from build123d import *

# Parameters (mm, degrees)
ESQUISSE1_R                                = 30
BOSS_EXTRU_1_DEPTH                         = 15
ESQUISSE2_R                                = 12.5
BOSS_EXTRU_2_DEPTH                         = 124
ESQUISSE4_2_W                              = 230
ESQUISSE4_2_H                              = 40
ENL_V_MAT_EXTRU_1_DEPTH                    = 5
CHAMBRAGE_POUR_VIS_T_TE_HEXAGONALE_2_COUNT = 2
CHAMBRAGE_POUR_VIS_T_TE_HEXAGONALE_2_PITCH = 41
ESQUISSE17_R                               = 6
BOSS_EXTRU_4_DEPTH                         = 83.38
ESQUISSE18_W                               = 10.356322474
ESQUISSE18_H                               = 3
ENL_V_MAT_EXTRU_2_DEPTH                    = 3
ESQUISSE19_W                               = 7.933443835
ESQUISSE19_H                               = 21.9317122
ENL_V_MAT_EXTRU_3_DEPTH                    = 50
BOSS_EXTRU_6_START                         = -10
ESQUISSE21_R                               = 12.5
BOSS_EXTRU_6_DEPTH                         = 10
D_GAGEMENT_M41_D                           = 4.5
D_GAGEMENT_M41_DEPTH                       = 3
D_GAGEMENT_M41_TIP                         = 1.299038106


with BuildPart() as part:
    # Esquisse1 → Boss.-Extru.1 (new body)
    with BuildSketch(Plane.XY):
        Circle(ESQUISSE1_R)
    extrude(amount=BOSS_EXTRU_1_DEPTH)

    # Esquisse2 → Boss.-Extru.2 (add)
    with BuildSketch(Plane(origin=(0, 0, 0), x_dir=(-1, 0, 0), z_dir=(0, 0, -1))):
        with Locations(Location((0, 0, 0), (0, 0, 180))):
            Circle(ESQUISSE2_R)
    extrude(amount=BOSS_EXTRU_2_DEPTH)

    # Esquisse4<2> → Enlèv. mat.-Extru.1 (cut)
    with BuildSketch(Plane.XY.offset(15)):
        Rectangle(ESQUISSE4_2_W, ESQUISSE4_2_H)
    extrude(amount=-ENL_V_MAT_EXTRU_1_DEPTH, mode=Mode.SUBTRACT)

    # Esquisse14 → Chambrage pour vis à tête hexagonale M51 (revolve, cut)
    with BuildSketch(Plane.YZ.offset(-20.5)):
        Polygon((0, 0), (0, 15), (2.75, 15), (2.75, 3.605), (2.775, 3.58), (6.12, 3.58), (6.12, 0), align=None)
    chambrage_pour_vis_t_te_hexagonale_m51 = revolve(axis=Axis((-20.5, 0, -6.35), (0, 0, 1)), mode=Mode.SUBTRACT)

    # Chambrage pour vis _ t_te hexagonale 2: Chambrage pour vis à tête hexagonale M51 ×2
    with Locations(*[(i * CHAMBRAGE_POUR_VIS_T_TE_HEXAGONALE_2_PITCH, 0, 0) for i in range(1, CHAMBRAGE_POUR_VIS_T_TE_HEXAGONALE_2_COUNT)]):
        add(chambrage_pour_vis_t_te_hexagonale_m51, mode=Mode.SUBTRACT)

    # Esquisse17 → Boss.-Extru.4 (add)
    with BuildSketch(Plane(origin=(0, 0, -124), x_dir=(-1, 0, 0), z_dir=(0, 0, -1))):
        Circle(ESQUISSE17_R)
    extrude(amount=BOSS_EXTRU_4_DEPTH)

    # Esquisse18 → Enlèv. mat.-Extru.2 (cut)
    with BuildSketch(Plane(origin=(0, 0, -207.38), x_dir=(-1, 0, 0), z_dir=(0, 0, -1))):
        with Locations((1.787207702, 0)):
            Rectangle(ESQUISSE18_W, ESQUISSE18_H)
    extrude(amount=-ENL_V_MAT_EXTRU_2_DEPTH, mode=Mode.SUBTRACT)

    # Esquisse19 → Enlèv. mat.-Extru.3 (cut)
    with BuildSketch(Plane(origin=(0, 0, -124), x_dir=(-1, 0, 0), z_dir=(0, 0, -1))):
        with Locations((9.966721917, 0)):
            Rectangle(ESQUISSE19_W, ESQUISSE19_H)
    extrude(amount=-ENL_V_MAT_EXTRU_3_DEPTH, mode=Mode.SUBTRACT)

    # Esquisse21 → Boss.-Extru.6 (add)
    with BuildSketch(Plane(origin=(0, 0, -124), x_dir=(-1, 0, 0), z_dir=(0, 0, -1)).offset(BOSS_EXTRU_6_START)):
        with Locations(Location((0, 0, 0), (0, 0, 180))):
            Circle(ESQUISSE21_R)
    extrude(amount=BOSS_EXTRU_6_DEPTH)

    # Dégagement M41
    with Locations(Plane.ZY.offset(6)):
        with Locations((-82.1, 5.85067254), (-93.1, -2.14932746), (-93.1, 5.85067254), (-104.1, 5.85067254)):
            Hole(D_GAGEMENT_M41_D / 2, depth=D_GAGEMENT_M41_DEPTH)
            with Locations((0, 0, -(D_GAGEMENT_M41_DEPTH + D_GAGEMENT_M41_TIP / 2))):  # 120° drill point
                Cone(0, D_GAGEMENT_M41_D / 2, D_GAGEMENT_M41_TIP, mode=Mode.SUBTRACT)


solid = part.part
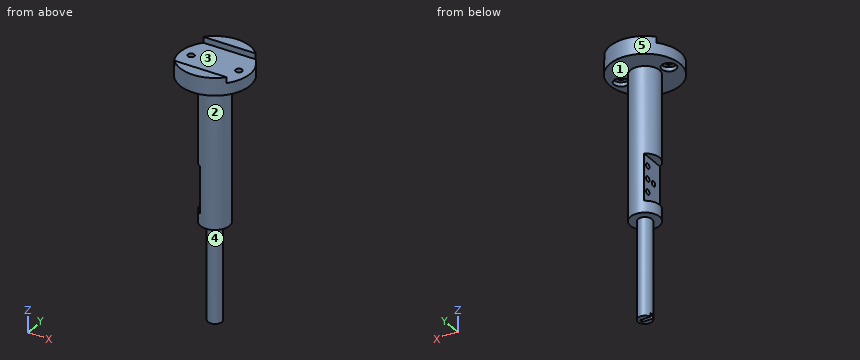
Design review of the part built by this model. Coordinates are the model's own, in mm. Face numbers are marked on the shaded views. A direction names the side the tool comes from. Coordinates: 2 decimals unless noted, no trailing zeros. Write each loop counter-clockwise with the first axis right and the second up, starting at its lowest first coordinate (ties: lowest second). Pieces come first, ordered by that corner, then holes. Notation, with made-up numbers: (-9.75, 16) -> (28.25, 16) arc R13 ccw to (28.25, 37) -> close; hole circle Ø7 at (49, -24). An arc over 180 degrees is marked (long way). Write each question's results on one line, items separated by ' | '. Start each with the question number.
(1) Take a section at C-C on y = 26.5. Write out the cut boundary in (x, z).
(2) Tool access review of the marked faces 4 and 5: name each direction out of +Z, -Z, +X, -X, +Y, -Y from which nothing blocks a thin tool from reaching the whole face with its end or side.
(3) For line 1 along X through (y, z) = (0, 2.2); line 2 along Y through (x, z) = (20, 5); line 3 along X through (y, z) = (0, 6), list the stretches that pass through material, from the lowest coordinate up. Write a range as from..to.
(4) Clearance check with flat-ended pins moving along their axes: P1, Ø0.9, axis at x = -3, z = -205.5, coming from the -Y side; P2, Ø4, axis at x = 5.5, z = -84.5, coming from the +Y side; P3, Ø6.5, axis at x = -20.5, y = 0, coming from the +Z side; P4, Ø6, axis at x = -14.5, y = 18, coming from the +Z side. State where each tip first meets the part, or that it passes through.
(5) Take a section at A-A on x = 1. Write out the cut boundary in (y, z).
(6) Take a section at B-B on z = -88.5. Write out the cut boundary in (x, y), and give its area (3 significant figures).
(7) The part is to be moulded in two halves that separate along Y. For the marked faces 1, 2 and 3, say which applies: pulls with the +Y half, pulls with the -Y half, needs draft (parallel to the pull), parting line crosses it, or undercut.
(8) Take a section at D-D on z = -173. Write out the cut boundary in (x, y).
Results found:
1) outline: (-14.06, 0) -> (14.06, 0) -> (14.06, 15) -> (-14.06, 15) -> close
2) face 4: -Z | face 5: +Z, -Z
3) line 1: x = -30..-26.62, -14.38..14.38, 26.62..30 | line 2: y = -22.36..-2.7, 2.7..22.36 | line 3: x = -30..-23.25, -17.75..17.75, 23.25..30
4) P1: stops at y = -5.43 | P2: stops at y = 12 | P3: stops at z = 10 | P4: stops at z = 15
5) outline: (-29.98, 0) -> (-12.46, 0) -> (-12.46, -124) -> (-5.92, -124) -> (-5.92, -207.38) -> (-1.5, -207.38) -> (-1.5, -204.38) -> (1.5, -204.38) -> (1.5, -207.38) -> (5.92, -207.38) -> (5.92, -124) -> (12.46, -124) -> (12.46, 0) -> (29.98, 0) -> (29.98, 15) -> (20, 15) -> (20, 10) -> (-20, 10) -> (-20, 15) -> (-29.98, 15) -> close
6) outline: (-6, -10.97) arc R12.5 ccw (long way) to (-6, 10.97) -> close | area: 389 mm2
7) face 1: needs draft | face 2: parting line crosses it | face 3: undercut
8) outline: circle Ø12 at (0, 0)
